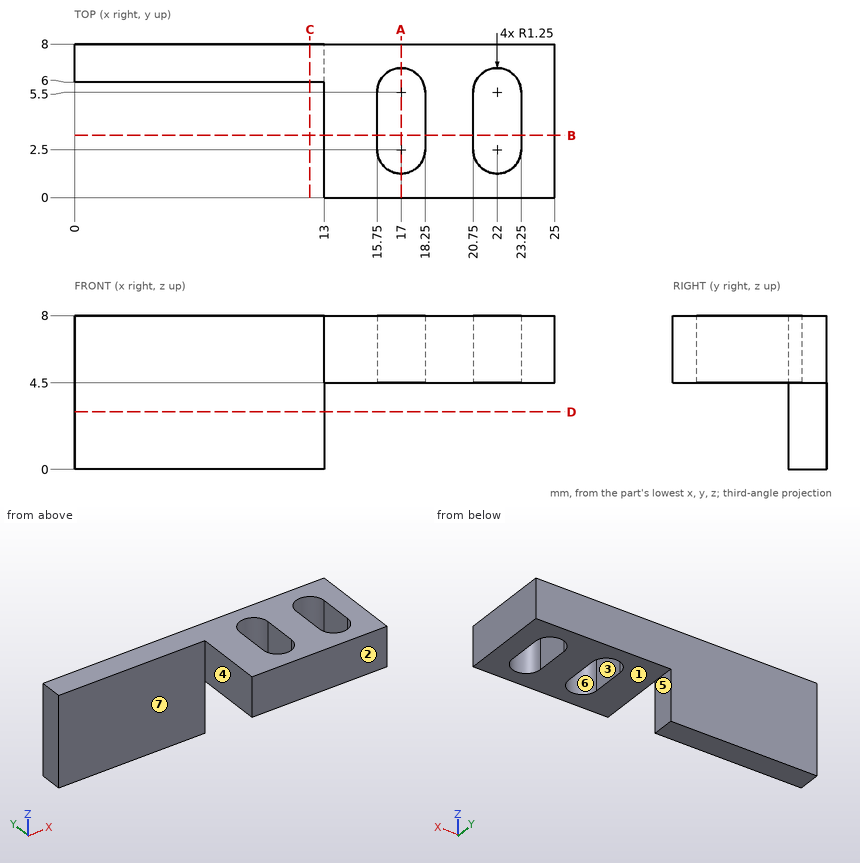
Answer from the drawing. Dimensions are ordinates in mm from the lowest x, y and z of the part. A direction names the side the tool comes from. Round coordinates to 2 decimals unless told otherwise and drop trailing zeros. Loops run counter-clockwise (first coordinate to the right, second up) from the corner with the lowest first, then second, coordinate; pieces in that order, holes last.
Q1. Section A-A on x = 17 is taken. Write down the section's boundary in (y, z), and give its area (3 significant figures).
Q2. Which of the six approach directions +Z, -Z, +X, -X, +Y, -Y give full straight-line access (tool end or side, diameter ignored) to the marked faces 1, 2, 3 and 4?
Q3. Section D-D on z = 3 is taken. Write down the section's boundary in (x, y).
Q4. Consider probe 1 along X at (y, z) = (2.5, 6.25); probe 2 along Y at (x, z) = (17, 5); probe 3 along X at (y, z) = (6.5, 6.75). Determine where each line is inside the solid, lowest interval first.
Q5. Each of these flat-tipped pins is pushed along its axis until it touches: pin 1 (1 mm diameter, centred on y = 7, z = 2, fed in from +X); pin 2 (0.9 mm diameter, centred on y = 3.5, z = 6.5, fed in from -X); pin 3 (4 mm diameter, centred on x = 16, y = 2.5, fed in from -Z). Where does it stop, or does it pass through?
Q6. Section B-B on y = 3.25 is taken. Write down the section's boundary in (x, z).
Q7. Section C-C on x = 12.25 is taken. Write down the section's boundary in (y, z), and give its area (3 significant figures).
Q8. Determine the mould class of the marked faces 5, 6 and 7 for opening direction X: released by +X, released by -X, zero draft, split by the parting line, or undercut.
Output:
1. outline: (0, 4.5) - (1.25, 4.5) - (1.25, 8) - (0, 8) - close; (6.75, 4.5) - (8, 4.5) - (8, 8) - (6.75, 8) - close
1. area: 8.75 mm2
2. face 1: -Z, +X, +Y, -Y
2. face 2: +Z, -Z, +X, -X, -Y
2. face 3: +Z, -Z
2. face 4: +Z, -Z, -X, -Y
3. outline: (0, 6) - (13, 6) - (13, 8) - (0, 8) - close
4. probe 1: x = 13 to 15.75, 18.25 to 20.75, 23.25 to 25
4. probe 2: y = 0 to 1.25, 6.75 to 8
4. probe 3: x = 0 to 16.25, 17.75 to 21.25, 22.75 to 25
5. pin 1: stops at x = 13
5. pin 2: stops at x = 13
5. pin 3: stops at z = 4.5
6. outline: (13, 4.5) - (15.75, 4.5) - (15.75, 8) - (13, 8) - close; (18.25, 4.5) - (20.75, 4.5) - (20.75, 8) - (18.25, 8) - close; (23.25, 4.5) - (25, 4.5) - (25, 8) - (23.25, 8) - close
7. outline: (6, 0) - (8, 0) - (8, 8) - (6, 8) - close
7. area: 16.0 mm2
8. face 5: released by +X
8. face 6: undercut
8. face 7: zero draft
